```python
from build123d import *

# Parameters (mm, degrees)
BOSS_EXTRUDE1_DEPTH      = 7
BOSS_EXTRUDE1_DEPTH_BACK = 7
FILLET1_R                = 10
SKETCH2_R                = 1
CUT_EXTRUDE1_DEPTH       = 45.028399926
SKETCH3_R                = 1.5
CUT_EXTRUDE2_DEPTH       = 5
SKETCH4_W                = 14
SKETCH4_H                = 8
SKETCH4_R                = 1.5
BOSS_EXTRUDE2_DEPTH      = 3


with BuildPart() as part:
    # Sketch1 → Boss-Extrude1 (new, two sides: drawn at the far end of the back side and taken through both)
    with BuildSketch(Plane(origin=(0, 0, 0), x_dir=(0, 0, -1), z_dir=(1, 0, 0)).offset(-BOSS_EXTRUDE1_DEPTH_BACK)):
        Polygon((-27, 0), (27, 0), (27, -23.5), (34.5, -23.5), (34.5, 7.5), (-34.5, 7.5), (-34.5, -23.5), (-27, -23.5), align=None)
    extrude(amount=BOSS_EXTRUDE1_DEPTH + BOSS_EXTRUDE1_DEPTH_BACK)

    # Fillet1
    fillet1_edges = [part.edges().sort_by_distance(p)[0] for p in [
        (0, 7.5, 34.5),
        (0, 7.5, -34.5),
    ]]
    fillet(fillet1_edges, radius=FILLET1_R)

    # Sketch2 → Cut-Extrude1 (cut, through all)
    with BuildSketch(Plane(origin=(7, 0, 0), x_dir=(0, 0, -1), z_dir=(1, 0, 0))):
        with Locations((-6.7, 2)):
            Circle(SKETCH2_R)
        with Locations((-20.1, 2)):
            Circle(SKETCH2_R)
        with Locations(Location((20.1, 2, 0), (0, 0, 180))):
            Circle(SKETCH2_R)
        with Locations(Location((6.7, 2, 0), (0, 0, 180))):
            Circle(SKETCH2_R)
    extrude(amount=-CUT_EXTRUDE1_DEPTH, mode=Mode.SUBTRACT)

    # Sketch3 → Cut-Extrude2 (cut)
    with BuildSketch(Plane.XZ.offset(23.5)):
        with Locations(Location((-3.5, -30.75, 0), (0, 0, 270))):
            Circle(SKETCH3_R)
        with Locations(Location((3.5, -30.75, 0), (0, 0, 90))):
            Circle(SKETCH3_R)
        with Locations(Location((-3.5, 30.75, 0), (0, 0, 90))):
            Circle(SKETCH3_R)
        with Locations(Location((3.5, 30.75, 0), (0, 0, 270))):
            Circle(SKETCH3_R)
    extrude(amount=-CUT_EXTRUDE2_DEPTH, mode=Mode.SUBTRACT)

    # Sketch4 → Boss-Extrude2 (add)
    # profile 1 of 2: a face of its own
    with BuildSketch(Plane.XZ.offset(23.5)):
        with Locations((0, 38.5)):
            Rectangle(SKETCH4_W, SKETCH4_H)
        with Locations(Location((-3.5, 39.5, 0), (0, 0, 270))):
            Circle(SKETCH4_R, mode=Mode.SUBTRACT)
        with Locations(Location((3.5, 39.5, 0), (0, 0, 90))):
            Circle(SKETCH4_R, mode=Mode.SUBTRACT)
    # profile 2 of 2: a face of its own
    with BuildSketch(Plane.XZ.offset(23.5)):
        with Locations((0, -38.5)):
            Rectangle(SKETCH4_W, SKETCH4_H)
        with Locations(Location((3.5, -39.5, 0), (0, 0, 270))):
            Circle(SKETCH4_R, mode=Mode.SUBTRACT)
        with Locations(Location((-3.5, -39.5, 0), (0, 0, 90))):
            Circle(SKETCH4_R, mode=Mode.SUBTRACT)
    extrude(amount=-BOSS_EXTRUDE2_DEPTH)


solid = part.part
```
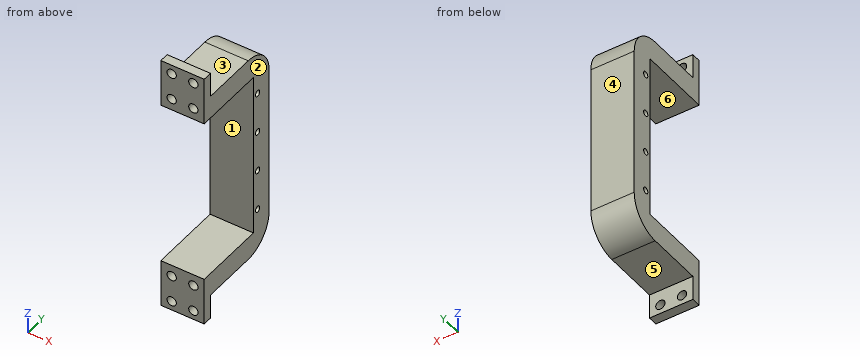
Design review of the part built by this model. Coordinates are the model's own, in mm. Face numbers are marked on the shaded views. A direction names the side the tool comes from. Coordinates: 2 decimals unless noted, no trailing zeros. Loops run counter-clockwise (first coordinate to the right, second up) from the corner with the lowest first, then second, coordinate; pieces in that order, holes last.
Q1. Tool access review of the marked faces 4, 5 and 6: name each direction out of +Z, -Z, +X, -X, +Y, -Y from which nothing blocks a thin tool from reaching the whole face with its end or side.
Reported:
face 4: +Z, -Z, +X, -X, +Y
face 5: -Z, +X, -X, +Y
face 6: +X, -X, -Y
Q2. We need section B-B on z = 6.7. State the section outline as (x, y) points.
Reported:
outline: (-7, 0) - (7, 0) - (7, 1) - (-7, 1) - close; (-7, 3) - (7, 3) - (7, 7.5) - (-7, 7.5) - close
Q3. We need section C-C on y = -8. State the section outline as (x, z) points.
Reported:
outline: (-7, -34.5) - (7, -34.5) - (7, -27) - (-7, -27) - close; (-7, 27) - (7, 27) - (7, 34.5) - (-7, 34.5) - close
Q4. To check wall thickness, follow line 1 (X direction, y = -20.85, z = 30.75); line 2 (Z direction, x = -1.5, y = -5.5); line 3 (Y direction, x = -3.25, z = -20.1). State the ranges of each line that lie inside material, in increasing order.
Reported:
line 1: x = -7 to -5, -2 to 2, 5 to 7
line 2: z = -34.5 to -27, 27 to 34.5
line 3: y = 0 to 1, 3 to 7.5
Q5. The part is to be moulded in two halves that separate along Z. For the marked faces 1, 2 and 3, say which applies: +Z half, -Z half, draft (parallel to the pull), parting line (faces both ways), or undercut.
Reported:
face 1: undercut
face 2: draft
face 3: +Z half
Q6. For pin 1 (8 mm diameter, centred on x = -3, y = -2, fed in from -Z); pin 2 (4 mm diameter, centred on x = 3, z = 7.5, fed in from -Y); pin 3 (1.5 mm diameter, centred on x = 3, z = 30.5, fed in from -Y); pin 4 (2.5 mm diameter, centred on x = 3.5, z = -39.5, fed in from +Y), all flat-tipped, find the tip position at first contact; note any pin that passes through.
Reported:
pin 1: stops at z = -34.5
pin 2: stops at y = 0
pin 3: stops at y = -18.5
pin 4: passes through
Q7. We need section D-D on z = -39.5. State the section outline as (x, y) points.
Reported:
outline: (-7, -23.5) - (-5, -23.5) - (-5, -20.5) - (-7, -20.5) - close; (-2, -23.5) - (2, -23.5) - (2, -20.5) - (-2, -20.5) - close; (5, -23.5) - (7, -23.5) - (7, -20.5) - (5, -20.5) - close
Q8. We need section A-A on x = -3.5. State how many separate pieces and enclosed holes the cut face has, and give its area (3 significant figures).
Reported:
separate pieces: 3
enclosed holes: 4
area: 815 mm2
